Design review of the part built by this model. Coordinates are the model's own, in mm. A direction names the side the tool comes from. Give positions to 0.01 mm unless a question says otherwise; leave off trailing zeros. Loops run counter-clockwise (first coordinate to the right, second up) from the corner with the lowest first, then second, coordinate; pieces in that order, holes last. Notation, with made-up numbers: (-25, 28) -> (13, 28) arc R20 cw to (13, 54) -> close; hole circle Ø2 at (38.25, 76.5). An arc over 180 degrees is marked (long way). Use CSV: the item, a comma, the result in double quotes. Start each with the question number.
Item 1: We need section B-B (x = 249). State the section outline as (y, z) points, plus the area to 3 significant figures.
Item 2: Clearance check with flat-ended pins moving along their axes: pin 1 (4 mm diameter, centred on x = 285.5, y = -8.5, fed in from +Z); pin 2 (8 mm diameter, centred on y = -12.5, z = 13.5, fed in from -X); pin 3 (1.5 mm diameter, centred on x = 277, z = 3.5, fed in from +Y); pin 4 (4 mm diameter, centred on x = 202, z = -15.5, fed in from +Y). State where each tip first meets the part, or that it passes through.
Item 3: Wall thickness on line 1 along Y through (x, z) = (318, 0); line 2 along X through (y, z) = (30, 22): over which ranges is each line inside the solid? List them lowest first. Write a range as from..to.
Item 4: The part is to be moulded in two halves that separate along X. For faces 6 (the face through (324, 0, 0)), 7 (the face through (-20.76, 9.76, -2.17)), 8 (the face through (311, 21, -28)), say which applies: +X half, -X half, draft (parallel to the pull), parting line (faces both ways), or undercut.
Item 5: We need section C-C (y = 31.5). State the section outline as (x, z) points.
Item 6: For faces 1 (the face through (-40, 0, 0)), 2 (the face through (144.942, -3.755, 11.923)), 3 (the face through (299, 35.4, 0.2)), 4 (the face through (296.46, 39.05, -8.67)), 5 (the face through (319.07, 19.524, -4.336)), list the 3-axis set-ups (+Z, -Z, +X, -X, +Y, -Y) from which the entire face can be reached by the end or side of a thin tool; tool diameter is ignored.
Item 7: We need section A-A (z = 28.5). State the section outline as (x, y) points, plus the area to 3 significant figures.
from build123d import *

# Parameters (mm, degrees)
F2_SIZE = 1
F3_SIZE = 1


# Not quite as in the source:
# - a feature names something its author has since deleted; it is built from what else it names


with BuildPart() as f1:
    # F0 (on Front) → F1 (revolve)
    with BuildSketch(Plane.XZ):
        Polygon((294, 12.5), (0, 12.5), (0, 7.5), (-2, 7.5), (-2, 10), (-40, 10), (-40, 0), (324, 0), (324, 12.5), (314, 12.5), (314, 20), (324, 20), (324, 40), (314, 40), (314, 35), (309, 35), (309, 40), (304, 40), (304, 35), (299, 35), (299, 40), (294, 40), align=None)
    revolve(axis=Axis((142, 0, 0), (1, 0, 0)))

    # F2
    f2_edges = [f1.edges().sort_by_distance(p)[0] for p in [
        (-2, 0, -7.5),
        (-40, 0, -10),
    ]]
    chamfer(f2_edges, length=F2_SIZE)

    # F3
    f3_edges = [f1.edges().sort_by_distance(p)[0] for p in [
        (324, 0, -12.5),
    ]]
    chamfer(f3_edges, length=F3_SIZE)


solid = f1.part
Results found:
1,outline,"circle Ø25 at (0, 0)"
1,area,"491 mm²"
2,pin 1,"z = 10.68"
2,pin 2,"x = 294"
2,pin 3,"y = 12.19"
2,pin 4,"through"
3,line 1,"-40..-20, -12.5..12.5, 20..40"
3,line 2,"294..299, 304..309, 314..324"
4,face 6,"+X half"
4,face 7,"draft"
4,face 8,"undercut"
5,outline,"(294, -24.65) -> (299, -24.65) -> (299, -15.26) -> (304, -15.26) -> (304, -24.65) -> (309, -24.65) -> (309, -15.26) -> (314, -15.26) -> (314, -24.65) -> (324, -24.65) -> (324, 24.65) -> (314, 24.65) -> (314, 15.26) -> (309, 15.26) -> (309, 24.65) -> (304, 24.65) -> (304, 15.26) -> (299, 15.26) -> (299, 24.65) -> (294, 24.65) -> close"
6,face 1,"+Z, -Z, -X, +Y, -Y"
6,face 2,"-X"
6,face 3,"none"
6,face 4,"+X, -X"
6,face 5,"+X"
7,outline,"(294, -28.07) -> (299, -28.07) -> (299, -20.32) -> (304, -20.32) -> (304, -28.07) -> (309, -28.07) -> (309, -20.32) -> (314, -20.32) -> (314, -28.07) -> (324, -28.07) -> (324, 28.07) -> (314, 28.07) -> (314, 20.32) -> (309, 20.32) -> (309, 28.07) -> (304, 28.07) -> (304, 20.32) -> (299, 20.32) -> (299, 28.07) -> (294, 28.07) -> close"
7,area,"1,530 mm²"
